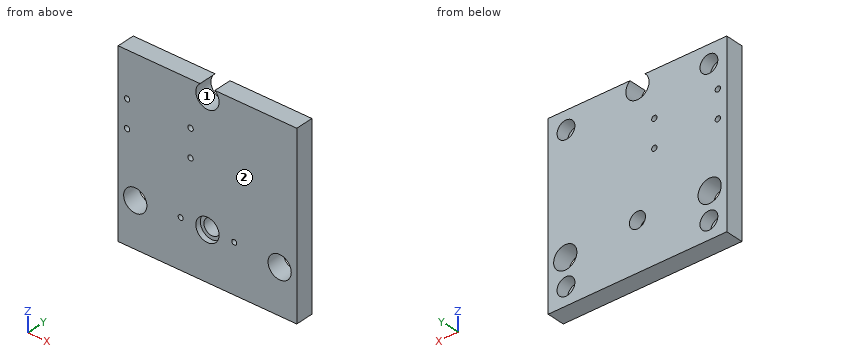
```python
from build123d import *

# Parameters (mm, degrees)
SKETCH_1_W          = 100
SKETCH_1_H          = 100
EXTRUDE_1_DEPTH     = 10
SKETCH_2_R          = 5
CUT_EXTRUDE_1_DEPTH = 7
SKETCH_3_R          = 6.5
CUT_EXTRUDE_2_DEPTH = 142.774468788
SKETCH_4_R          = 4.5
CUT_EXTRUDE_3_DEPTH = 142.774468788
SKETCH_5_R          = 6.5
CUT_EXTRUDE_4_DEPTH = 3
SKETCH_6_R          = 1.5
CUT_EXTRUDE_5_DEPTH = 142.774468788
SKETCH_7_R          = 1.4
CUT_EXTRUDE_6_DEPTH = 5


with BuildPart() as part:
    # 草图1 → 凸台-拉伸1 (new body)
    with BuildSketch(Plane(origin=(0, 0, 0), x_dir=(1, 0, 0), z_dir=(0, 1, 0))):
        with Locations((50, -50)):
            Rectangle(SKETCH_1_W, SKETCH_1_H)
    extrude(amount=EXTRUDE_1_DEPTH)

    # 草图2 → 切除-拉伸1 (cut)
    with BuildSketch(Plane(origin=(0, 10, 0), x_dir=(1, 0, 0), z_dir=(0, 1, 0))):
        with Locations(Location((10, -10, 0), (0, 0, 270))):
            Circle(SKETCH_2_R)
        with Locations(Location((90, -10, 0), (0, 0, 270))):
            Circle(SKETCH_2_R)
        with Locations(Location((10, -90, 0), (0, 0, 270))):
            Circle(SKETCH_2_R)
        with Locations(Location((90, -90, 0), (0, 0, 270))):
            Circle(SKETCH_2_R)
    extrude(amount=-CUT_EXTRUDE_1_DEPTH, mode=Mode.SUBTRACT)

    # 草图3 → 切除-拉伸2 (cut, through all)
    with BuildSketch(Plane(origin=(0, 10, 0), x_dir=(1, 0, 0), z_dir=(0, 1, 0))):
        with Locations((50, -95)):
            Circle(SKETCH_3_R)
        with Locations(Location((90.414518843, -25, 0), (0, 0, 270))):
            Circle(SKETCH_3_R)
        with Locations(Location((9.585481157, -25, 0), (0, 0, 270))):
            Circle(SKETCH_3_R)
    extrude(amount=-CUT_EXTRUDE_2_DEPTH, mode=Mode.SUBTRACT)

    # 草图4 → 切除-拉伸3 (cut, through all)
    with BuildSketch(Plane(origin=(0, 10, 0), x_dir=(1, 0, 0), z_dir=(0, 1, 0))):
        with Locations(Location((50, -27, 0), (0, 0, 270))):
            Circle(SKETCH_4_R)
    extrude(amount=-CUT_EXTRUDE_3_DEPTH, mode=Mode.SUBTRACT)

    # 草图5 → 切除-拉伸4 (cut)
    with BuildSketch(Plane(origin=(0, 0, 0), x_dir=(-1, 0, 0), z_dir=(0, -1, 0))):
        with Locations(Location((-50, -27, 0), (0, 0, 90))):
            Circle(SKETCH_5_R)
    extrude(amount=-CUT_EXTRUDE_4_DEPTH, mode=Mode.SUBTRACT)

    # 草图6 → 切除-拉伸5 (cut, through all)
    with BuildSketch(Plane(origin=(0, 10, 0), x_dir=(1, 0, 0), z_dir=(0, 1, 0))):
        with Locations(Location((40.56, -59.76, 0), (0, 0, 270))):
            Circle(SKETCH_6_R)
        with Locations(Location((40.56, -75, 0), (0, 0, 270))):
            Circle(SKETCH_6_R)
        with Locations(Location((5, -59.76, 0), (0, 0, 270))):
            Circle(SKETCH_6_R)
        with Locations(Location((5, -75, 0), (0, 0, 270))):
            Circle(SKETCH_6_R)
    extrude(amount=-CUT_EXTRUDE_5_DEPTH, mode=Mode.SUBTRACT)

    # 草图7 → 切除-拉伸6 (cut)
    with BuildSketch(Plane(origin=(0, 0, 0), x_dir=(-1, 0, 0), z_dir=(0, -1, 0))):
        with Locations(Location((-65, -27, 0), (0, 0, 90))):
            Circle(SKETCH_7_R)
        with Locations(Location((-35, -27, 0), (0, 0, 90))):
            Circle(SKETCH_7_R)
    extrude(amount=-CUT_EXTRUDE_6_DEPTH, mode=Mode.SUBTRACT)


solid = part.part
```
Source: CAD feature listing. Evaluate the final solid. Frame: model axes, mm. Face numbers are marked on the shaded views. Give positions to 0.01 mm unless a question says otherwise; leave off trailing zeros. Loops run counter-clockwise (first coordinate to the right, second up) from the corner with the lowest first, then second, coordinate; pieces in that order, holes last. Notation, with made-up numbers: (-2, 11.5) - (3, 11.5) arc R28 ccw to (3, 46.5) - close; hole circle Ø1 at (-7.75, 43.5). An arc over 180 degrees is marked (long way). Use CSV: the item, a comma, the result in double quotes. Start each with the question number.
1. Draft query along X for the marked faces 1 and 2. Return one class per face: +X half, -X half, draft (parallel to the pull), parting line (faces both ways), or undercut.
2. Section A-A (x = 50). Output: boundary loops of the cut face in (y, z), then the cut area to 3 significant figures.
3. Ray query, L1, parallel to X at y = 4.25, z = 59.76; L2, parallel to X at y = 8.5, z = 90; L3, parallel to Z at x = 65, y = 3.55. Return the intervals inside material, ascending.
4. Section D-D (z = 27). Output: boundary loops of the cut face in (x, y).
5. Pin query (flat end, axial travel): pin 1 (10.5 mm diameter, centred on x = 50, z = 27, fed in from -Y); pin 2 (2.5 mm diameter, centred on x = 35, z = 27, fed in from -Y); pin 3 (8 mm diameter, centred on x = 50, z = 27, fed in from -Y). Return the tip coordinate at first contact, or that it passes through.
6. Section C-C (y = 7). Count the separate pieces of the cut face and the enclosed holes in it, then the cut area to 3 significant figures.
7. Section B-B (z = 75). Output: boundary loops of the cut face in (x, y).
Response:
1,face 1,"undercut"
1,face 2,"draft"
2,outline,"(0, 0) - (10, 0) - (10, 22.5) - (3, 22.5) - (3, 20.5) - (0, 20.5) - close; (0, 33.5) - (3, 33.5) - (3, 31.5) - (10, 31.5) - (10, 88.5) - (0, 88.5) - close"
2,area,"783 mm²"
3,L1,"0 to 3.5, 6.5 to 39.06, 42.06 to 100"
3,L2,"0 to 5, 15 to 45.85, 54.15 to 85, 95 to 100"
3,L3,"0 to 25.6, 28.4 to 100"
4,outline,"(0, 0) - (3.4, 0) - (3.4, 10) - (0, 10) - close; (15.77, 0) - (33.6, 0) - (33.6, 5) - (36.4, 5) - (36.4, 0) - (43.5, 0) - (43.5, 3) - (45.5, 3) - (45.5, 10) - (15.77, 10) - close; (54.5, 3) - (56.5, 3) - (56.5, 0) - (63.6, 0) - (63.6, 5) - (66.4, 5) - (66.4, 0) - (84.23, 0) - (84.23, 10) - (54.5, 10) - close; (96.6, 0) - (100, 0) - (100, 10) - (96.6, 10) - close"
5,pin 1,"y = 3"
5,pin 2,"y = 5"
5,pin 3,"through"
6,separate pieces,"1"
6,enclosed holes,"11"
6,area,"9,200 mm²"
7,outline,"(0, 0) - (3.5, 0) - (3.5, 10) - (0, 10) - close; (6.5, 0) - (39.06, 0) - (39.06, 10) - (6.5, 10) - close; (42.06, 0) - (100, 0) - (100, 10) - (42.06, 10) - close"
